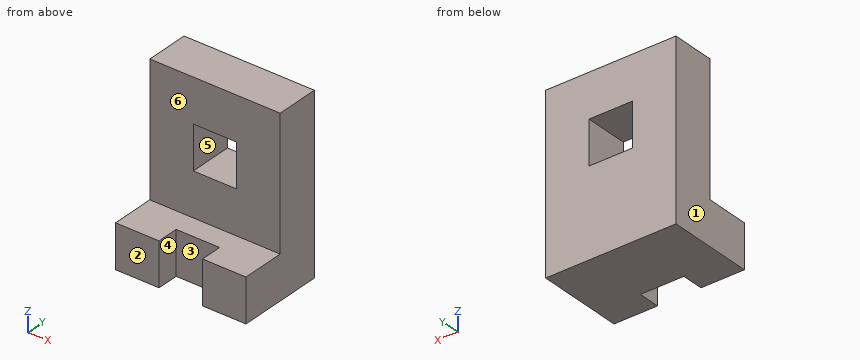
from build123d import *

# Parameters (mm, degrees)
F0_W     = 25.4
F0_H     = 25.4
F1_DEPTH = 38.1
F2_DEPTH = 12.7
F3_DEPTH = 25.4
F4_DEPTH = 12.7
F5_DEPTH = 12.7


with BuildPart() as f1:
    # F0 (on Front) → F1 (new body)
    with BuildSketch(Plane.XZ):
        with Locations((-25.4, -13.468404)):
            Rectangle(F0_W, F0_H)
        with Locations((25.4, -13.468404)):
            Rectangle(F0_W, F0_H)
    extrude(amount=F1_DEPTH)

    # F0 (on Front) → F2 (join)
    with BuildSketch(Plane.XZ):
        with Locations((25.4, -13.468404)):
            Rectangle(F0_W, F0_H)
        with Locations((-25.4, -13.468404)):
            Rectangle(F0_W, F0_H)
    extrude(amount=-F2_DEPTH)

    # F0 (on Front) → F3 (join)
    with BuildSketch(Plane.XZ):
        with Locations((0, -13.468404)):
            Rectangle(F0_W, F0_H)
    extrude(amount=F3_DEPTH)

    # F0 (on Front) → F4 (join)
    with BuildSketch(Plane.XZ):
        with Locations((0, -13.468404)):
            Rectangle(F0_W, F0_H)
    extrude(amount=-F4_DEPTH)

    # F0 (on Front) → F5 (join, symmetric)
    with BuildSketch(Plane.XZ):
        Polygon((38.1, 75.431596), (-38.1, 75.431596), (-38.1, -0.768404), (-12.7, -0.768404), (12.7, -0.768404), (38.1, -0.768404), align=None)
        with Locations((0, 37.331596)):
            Rectangle(F0_W, F0_H, mode=Mode.SUBTRACT)
    extrude(amount=F5_DEPTH, both=True)


solid = f1.part
Read the model definition and answer for the solid it produces. Units are mm, in the model's axes. Face numbers are marked on the shaded views. A direction names the side the tool comes from. Coordinates: 2 decimals unless noted, no trailing zeros. Order: outer loops, then holes, each group sorted by start corner. A loop starts at its lowest first (then second) coordinate and runs counter-clockwise, first axis right, second up. Notation, with made-up numbers: M -25,72.25 L 25,72.25 A17 ccw 25,94.25 Z; hole C -20,42.5 d2. An arc over 180 degrees is marked long. Put each result on its own line as item: value. Start each with the question number.
Item 1: Section A-A, the plane x = -4.5 is taken. Determine the outline of the cut face in (y, z), plus the area to 3 significant figures.
Item 2: Consider probe 1 along X at (y, z) = (-0.5, 33); probe 2 along Z at (x, y) = (-3, 9); probe 3 along Y at (x, z) = (20, 67). Determine where each line is inside the solid, lowest interval first. Write a range as [from, to].
Item 3: Given pin 1 Ø8 at (x, z) = (-2, 64.5) entering from -Y; pin 2 Ø12.5 at (x, z) = (0, -14.5) entering from -Y; pin 3 Ø1.5 at (x, y) = (14.5, -28.5) entering from +Z, each flat-ended and moving along its own axis, determine where each tip first touches the part or whether it passes through.
Item 4: Section B-B, the plane y = -33.5 is taken. Determine the outline of the cut face in (x, z), plus the area to 3 significant figures.
Item 5: Section C-C, the plane z = -8.5 is taken. Determine the outline of the cut face in (x, y), plus the area to 3 significant figures.
Item 6: For the marked faces 4, 5 and 6, determine the directions among +Z, -Z, +X, -X, +Y, -Y from which every point of the face is accessible in a straight line to the end or side of a thin tool.
Item 7: Section D-D, the plane y = 8 is taken. Determine the outline of the cut face in (x, z), plus the area to 3 significant figures.
Item 8: The mould has two halves that part along X. Classify the marked faces 1, 2 and 3: +X half, -X half, draft (parallel to the pull), parting line (faces both ways), or undercut.
Computed:
1. outline: M -25.4,-26.17 L 12.7,-26.17 L 12.7,24.63 L -12.7,24.63 L -12.7,-0.77 L -25.4,-0.77 Z; M -12.7,50.03 L 12.7,50.03 L 12.7,75.43 L -12.7,75.43 Z
1. area: 2,260 mm2
2. probe 1: x = [-38.1, -12.7], [12.7, 38.1]
2. probe 2: z = [-26.17, 24.63], [50.03, 75.43]
2. probe 3: y = [-12.7, 12.7]
3. pin 1: stops at y = -12.7
3. pin 2: stops at y = -25.4
3. pin 3: stops at z = -0.77
4. outline: M -38.1,-26.17 L -12.7,-26.17 L -12.7,-0.77 L -38.1,-0.77 Z; M 12.7,-26.17 L 38.1,-26.17 L 38.1,-0.77 L 12.7,-0.77 Z
4. area: 1,290 mm2
5. outline: M -38.1,-38.1 L -12.7,-38.1 L -12.7,-25.4 L 12.7,-25.4 L 12.7,-38.1 L 38.1,-38.1 L 38.1,12.7 L -38.1,12.7 Z
5. area: 3,550 mm2
6. face 4: +Z, -Z, -Y
6. face 5: +Y, -Y
6. face 6: +Z, +X, -X, -Y
7. outline: M -38.1,-26.17 L 38.1,-26.17 L 38.1,75.43 L -38.1,75.43 Z; hole M -12.7,24.63 L 12.7,24.63 L 12.7,50.03 L -12.7,50.03 Z
7. area: 7,100 mm2
8. face 1: -X half
8. face 2: draft
8. face 3: undercut
